Print and shaded views of the part. All mm, measured from the part's lowest x, y and z. Give positions to 0.01 mm unless a question says otherwise; leave off trailing zeros. Loops run counter-clockwise (first coordinate to the right, second up) from the corner with the lowest first, then second, coordinate; pieces in that order, holes last. Notation, with made-up numbers: M 78.5,38 L 82.5,38 A9 ccw 82.5,50 Z; hole C 55,14.25 d7. An arc over 180 degrees is marked long. Answer in a Markdown table with one row per item.
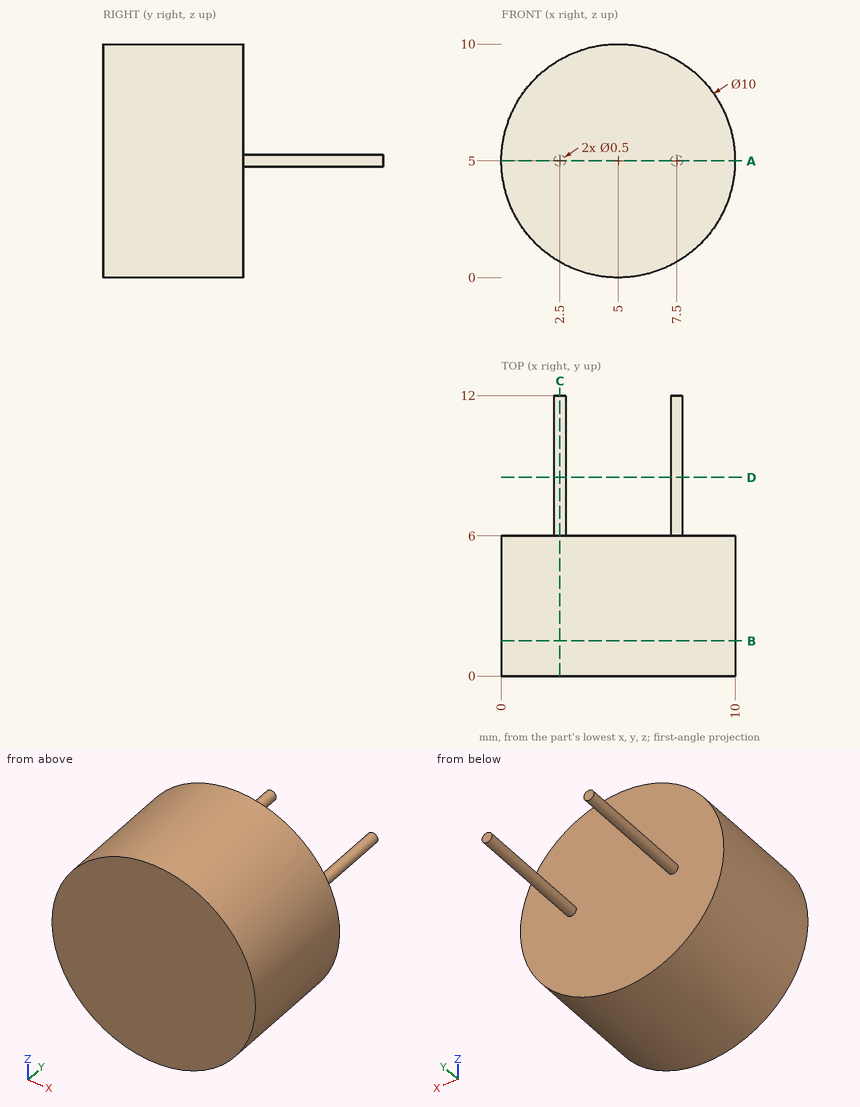
(1) Wall check: L1, parallel to Y at x = 1.75, z = 6.75; L2, parallel to X at y = 3.75, z = 3.5; L3, parallel to X at y = 2.75, z = 3.25. Give the ranges that are in metal, low to high.
Established:
| item | result |
|---|---|
| L1 | y = 0 to 6 |
| L2 | x = 0.23 to 9.77 |
| L3 | x = 0.32 to 9.68 |
(2) Saw through at C-C, the plane x = 2.5. Give the cut face in (y, z).
Established:
| item | result |
|---|---|
| outline | M 0,0.67 L 6,0.67 L 6,4.75 L 12,4.75 L 12,5.25 L 6,5.25 L 6,9.33 L 0,9.33 Z |
(3) Flat gauge pins, fed straight in: P1, Ø2, axis at x = 4.5, z = 1.5, coming from the +Y side; P2, Ø4, axis at y = 9, z = 3, coming from the -X side; P3, Ø1.5, axis at y = 6, z = 3, coming from the -X side. Where does each tip first touch, or does it go through?
Established:
| item | result |
|---|---|
| P1 | stops at y = 6 |
| P2 | stops at x = 2.25 |
| P3 | stops at x = 0.16 |
(4) Saw through at D-D, the plane y = 8.5. Give the cut face in (x, z), and give its area (3 significant figures).
Established:
| item | result |
|---|---|
| outline | C 2.5,5 d0.5; C 7.5,5 d0.5 |
| area | 0.393 mm2 |
(5) Saw through at A-A, the plane z = 5. Give the cut face in (x, y), and give its area (3 significant figures).
Established:
| item | result |
|---|---|
| outline | M 0,0 L 10,0 L 10,6 L 7.75,6 L 7.75,12 L 7.25,12 L 7.25,6 L 2.75,6 L 2.75,12 L 2.25,12 L 2.25,6 L 0,6 Z |
| area | 66.0 mm2 |
(6) Saw through at B-B, the plane y = 1.5. Give the cut face in (x, z), and give its area (3 significant figures).
Established:
| item | result |
|---|---|
| outline | C 5,5 d10 |
| area | 78.5 mm2 |
